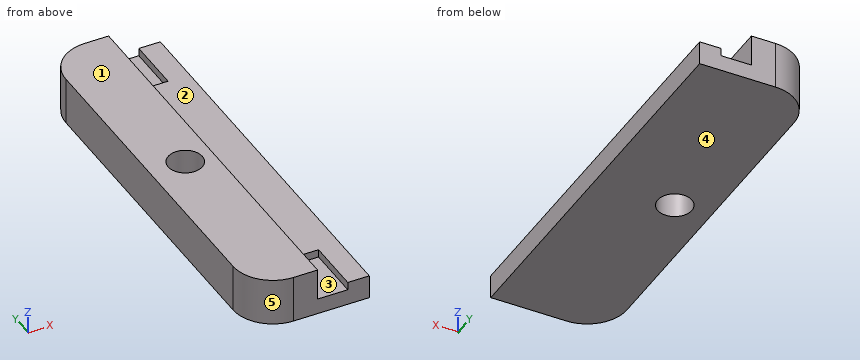
```python
from build123d import *

# Parameters (mm, degrees)
CROQUIS1_W              = 14.5
CROQUIS1_H              = 50
CROQUIS1_R              = 2.15
SALIENTE_EXTRUIR1_DEPTH = 6
CROQUIS3_W              = 6.5
CROQUIS3_H              = 3
CORTAR_EXTRUIR1_DEPTH   = 50
CROQUIS4_W              = 3.8
CROQUIS4_H              = 1
CORTAR_EXTRUIR2_DEPTH   = 7
CORTAR_EXTRUIR3_START   = -50
CROQUIS4_2_W            = 3.8
CROQUIS4_2_H            = 1
CORTAR_EXTRUIR3_DEPTH   = 7
REDONDEO1_R             = 5


with BuildPart() as part:
    # Croquis1 → Saliente-Extruir1 (new body)
    with BuildSketch(Plane.XY):
        with Locations((2.75, 0)):
            Rectangle(CROQUIS1_W, CROQUIS1_H)
        Circle(CROQUIS1_R, mode=Mode.SUBTRACT)
    extrude(amount=SALIENTE_EXTRUIR1_DEPTH)

    # Croquis3 → Cortar-Extruir1 (cut)
    with BuildSketch(Plane.XZ.offset(25)):
        with Locations((6.75, 4.5)):
            Rectangle(CROQUIS3_W, CROQUIS3_H)
    extrude(amount=-CORTAR_EXTRUIR1_DEPTH, mode=Mode.SUBTRACT)

    # Croquis4 → Cortar-Extruir2 (cut)
    with BuildSketch(Plane(origin=(0, 25, 0), x_dir=(1, 0, 0), z_dir=(0, 1, 0))):
        with Locations((5.4, -2.5)):
            Rectangle(CROQUIS4_W, CROQUIS4_H)
    extrude(amount=-CORTAR_EXTRUIR2_DEPTH, mode=Mode.SUBTRACT)

    # Croquis4<2> → Cortar-Extruir3 (cut)
    with BuildSketch(Plane(origin=(0, 25, 0), x_dir=(1, 0, 0), z_dir=(0, 1, 0)).offset(CORTAR_EXTRUIR3_START)):
        with Locations((5.4, -2.5)):
            Rectangle(CROQUIS4_2_W, CROQUIS4_2_H)
    extrude(amount=CORTAR_EXTRUIR3_DEPTH, mode=Mode.SUBTRACT)

    # Redondeo1
    redondeo1_edges = [part.edges().sort_by_distance(p)[0] for p in [
        (-4.5, 25, 3),
        (-4.5, -25, 3),
    ]]
    fillet(redondeo1_edges, radius=REDONDEO1_R)


solid = part.part
```
The listing builds one solid part. Answer for the finished solid, in the listing's coordinates (mm). Face numbers are marked on the shaded views. A direction names the side the tool comes from. Round coordinates to 2 decimals unless told otherwise and drop trailing zeros. Write each loop counter-clockwise with the first axis right and the second up, starting at its lowest first coordinate (ties: lowest second). Pieces come first, ordered by that corner, then holes. Notation, with made-up numbers: (54.25, 36.5) -> (69.25, 36.5) arc R5 ccw to (69.25, 45.5) -> close; hole circle Ø5 at (35, 71.25). An arc over 180 degrees is marked (long way). Answer as a JSON object with one key per item and string values. Group by question number.
Q1. Each of these flat-tipped pins is pushed along its axis until it touches: pin 1 Ø4 at (x, y) = (0, 0) entering from +Z; pin 2 Ø3 at (x, z) = (-2.5, 4) entering from -Y; pin 3 Ø1.1 at (y, z) = (21.5, 2.5) entering from -X; pin 4 Ø1.1 at (x, y) = (5, -20.5) entering from +Z. Where does it stop, or does it pass through?
Q2. Section B-B (z = 0.5) is taken. Write down the section's boundary in (x, y).
Q3. Section C-C (x = 6.5) is taken. Write down the section's boundary in (y, z), plus the area to 3 significant figures.
Q4. Section A-A (y = 0) is taken. Write down the section's boundary in (x, z).
Q5. Determine the mould class of the marked faces 3, 4 and 5 for opening direction X: pulls with the +X half, pulls with the -X half, needs draft (parallel to the pull), parting line crosses it, or undercut.
Q6. Which of the six approach directions +Z, -Z, +X, -X, +Y, -Y give full straight-line access (tool end or side, diameter ignored) to the marked faces 1 and 2?
Q7. Straight lines are drawn through the part: line 1 along X through (y, z) = (-20, 2.75); line 2 along X through (y, z) = (-7, 5.45); line 3 along Y through (x, z) = (0, 2.35). For each, find the intervals that lie inside material, in ascending order.
Q8. Section D-D (y = -8.5) is taken. Write down the section's boundary in (x, z).
Check values:
{
 "1": {"pin 1": "through", "pin 2": "y = -24.77", "pin 3": "x = -4.41", "pin 4": "z = 2"},
 "2": {"outline": "(-4.5, -20) arc R5 ccw to (0.5, -25) -> (10, -25) -> (10, 25) -> (0.5, 25) arc R5 ccw to (-4.5, 20) -> close; hole circle Ø4.3 at (0, 0)"},
 "3": {"outline": "(-25, 0) -> (25, 0) -> (25, 2) -> (18, 2) -> (18, 3) -> (-18, 3) -> (-18, 2) -> (-25, 2) -> close", "area": "136 mm^2"},
 "4": {"outline": "(-4.5, 0) -> (-2.15, 0) -> (-2.15, 6) -> (-4.5, 6) -> close; (2.15, 0) -> (10, 0) -> (10, 3) -> (3.5, 3) -> (3.5, 6) -> (2.15, 6) -> close"},
 "5": {"face 3": "undercut", "face 4": "needs draft", "face 5": "pulls with the -X half"},
 "6": {"face 1": "+Z, +X, -X, +Y, -Y", "face 2": "+Z, +X, +Y, -Y"},
 "7": {"line 1": "-4.5 to 3.5, 7.3 to 10", "line 2": "-4.5 to 3.5", "line 3": "-24.97 to -2.15, 2.15 to 24.97"},
 "8": {"outline": "(-4.5, 0) -> (10, 0) -> (10, 3) -> (3.5, 3) -> (3.5, 6) -> (-4.5, 6) -> close"}
}
